from build123d import *

# Parameters (mm, degrees)
SKETCH_1_W          = 131
SKETCH_1_H          = 36
SKETCH_1_W_2        = 125
SKETCH_1_H_2        = 30
EXTRUDE_3_DEPTH     = 50
SKETCH_4_W          = 131
SKETCH_4_H          = 36
EXTRUDE_4_DEPTH     = 3
SKETCH_5_R          = 7.5
CUT_EXTRUDE_1_DEPTH = 3
CUT_EXTRUDE_2_DEPTH = 3
SKETCH_11_W         = 1
SKETCH_11_H         = 30
EXTRUDE_6_DEPTH     = 50
SKETCH_8_W          = 131
SKETCH_8_H          = 36
EXTRUDE_7_DEPTH     = 3
SKETCH_12_W         = 127.4
SKETCH_12_H         = 52.4
CUT_EXTRUDE_4_DEPTH = 3
CUT_EXTRUDE_5_DEPTH = 3
FILLET_5_R          = 3
FILLET_6_R          = 1


with BuildPart() as part:
    # 草图1 → 凸台-拉伸3 (new body)
    with BuildSketch(Plane.XY):
        with Locations((62.5, -15)):
            Rectangle(SKETCH_1_W, SKETCH_1_H)
        with Locations((62.5, -15)):
            Rectangle(SKETCH_1_W_2, SKETCH_1_H_2, mode=Mode.SUBTRACT)
    extrude(amount=EXTRUDE_3_DEPTH)

    # 草图4 → 凸台-拉伸4 (add)
    with BuildSketch(Plane(origin=(0, 0, 0), x_dir=(-1, 0, 0), z_dir=(0, 0, -1))):
        with Locations((-62.5, -15)):
            Rectangle(SKETCH_4_W, SKETCH_4_H)
    extrude(amount=EXTRUDE_4_DEPTH)

    # 草图5 → 切除-拉伸1 (cut)
    with BuildSketch(Plane(origin=(0, 3, 0), x_dir=(1, 0, 0), z_dir=(0, 1, 0))):
        with Locations(Location((17.5, -30, 0), (0, 0, 270))):
            Circle(SKETCH_5_R)
        with Locations(Location((47.5, -30, 0), (0, 0, 270))):
            Circle(SKETCH_5_R)
        with Locations(Location((77.5, -30, 0), (0, 0, 270))):
            Circle(SKETCH_5_R)
        with Locations(Location((107.5, -30, 0), (0, 0, 270))):
            Circle(SKETCH_5_R)
    extrude(amount=-CUT_EXTRUDE_1_DEPTH, mode=Mode.SUBTRACT)

    # 草图6 → 切除-拉伸2 (cut)
    with BuildSketch(Plane.XZ.offset(33)):
        Polygon((10, 25), (10, 27.5), (115, 27.5), (115, 25), (115, 22.5), (10, 22.5), align=None)
    extrude(amount=-CUT_EXTRUDE_2_DEPTH, mode=Mode.SUBTRACT)

    # 草图11 → 凸台-拉伸6 (add)
    with BuildSketch(Plane.XY.offset(50)):
        with Locations((0.5, -15)):
            Rectangle(SKETCH_11_W, SKETCH_11_H)
        with Locations((124.5, -15)):
            Rectangle(SKETCH_11_W, SKETCH_11_H)
    extrude(amount=-EXTRUDE_6_DEPTH)

    # 草图8 → 凸台-拉伸7 (add)
    with BuildSketch(Plane.XY.offset(50)):
        with Locations((62.5, -15)):
            Rectangle(SKETCH_8_W, SKETCH_8_H)
    extrude(amount=EXTRUDE_7_DEPTH)

    # 草图12 → 切除-拉伸4 (cut)
    with BuildSketch(Plane(origin=(0, 3, 0), x_dir=(1, 0, 0), z_dir=(0, 1, 0))):
        with Locations((62.5, -25)):
            Rectangle(SKETCH_12_W, SKETCH_12_H)
    extrude(amount=-CUT_EXTRUDE_4_DEPTH, mode=Mode.SUBTRACT)

    # 草图13 → 切除-拉伸5 (cut)
    with BuildSketch(Plane.XY.offset(53)):
        Polygon((47, -15), (47, -5), (78, -5), (78, -25), (47, -25), align=None)
    extrude(amount=-CUT_EXTRUDE_5_DEPTH, mode=Mode.SUBTRACT)

    # 圆角5
    fillet_5_edges = [part.edges().sort_by_distance(p)[0] for p in [
        (-3, -15, 53),
        (62.5, -33, 53),
        (128, -15, 53),
        (128, -15, -3),
        (62.5, -33, -3),
        (-3, -15, -3),
        (128, -33, 25),
        (-3, -33, 25),
    ]]
    fillet(fillet_5_edges, radius=FILLET_5_R)

    # 圆角6
    fillet_6_edges = [part.edges().sort_by_distance(p)[0] for p in [
        (47, -15, 50),
        (62.5, -5, 50),
        (78, -15, 50),
        (62.5, -25, 50),
        (47, -15, 53),
        (62.5, -25, 53),
        (78, -15, 53),
        (62.5, -5, 53),
    ]]
    fillet(fillet_6_edges, radius=FILLET_6_R)


solid = part.part
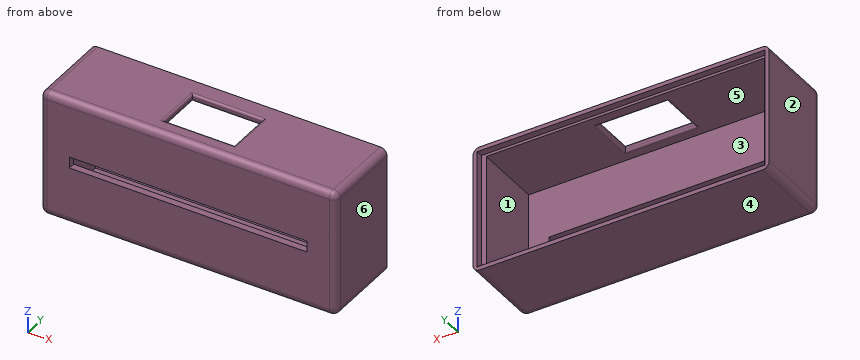
Can you work these out from the model? Positions are in its coordinate system, mm. Face numbers are marked on the shaded views. A direction names the side the tool comes from. Give positions to 0.01 mm unless a question says otherwise; leave off trailing zeros. Order: outer loops, then holes, each group sorted by start corner. A loop starts at its lowest first (then second) coordinate and runs counter-clockwise, first axis right, second up. Notation, with made-up numbers: M -37,48.25 L 14,48.25 A20 cw 14,77.25 Z; hole C 74,-26.75 d8. An arc over 180 degrees is marked long. Use one line per item in the form item = value.
Item 1: If we section it at A-A, the plane x = 64.5: Write out the boundary of the cut face in (y, z).
Values follow:
outline = M -33,0 A3 ccw -30,-3 L 3,-3 L 3,-1.2 L 0,-1.2 L 0,0 L -30,0 L -30,22.5 L -33,22.5 Z; M -33,27.5 L -30,27.5 L -30,50 L -26,50 A1 ccw -25,51 L -25,52 A1 ccw -26,53 L -30,53 A3 ccw -33,50 Z; M -5,51 A1 ccw -4,50 L 0,50 L 0,51.2 L 3,51.2 L 3,53 L -4,53 A1 ccw -5,52 Z
Item 2: For the marked faces 5 and 6, which set-ups out of +Z, -Z, +X, -X, +Y, -Y let a thin tool reach every point of the face, with its end or its side?
Values follow:
face_5 = +Y
face_6 = +Z, -Z, +X, +Y, -Y
Item 3: If we section it at C-C, the plane x = 24: Write out the boundary of the cut face in (y, z).
Values follow:
outline = M -33,0 A3 ccw -30,-3 L 3,-3 L 3,-1.2 L 0,-1.2 L 0,0 L -30,0 L -30,22.5 L -33,22.5 Z; M -33,27.5 L -30,27.5 L -30,50 L 0,50 L 0,51.2 L 3,51.2 L 3,53 L -30,53 A3 ccw -33,50 Z
Item 4: Will these pins go through, and if not, where does the flat tip stop? pin 1 Ø0.9 at (x, y) = (57, -32) entering from +Z; pin 2 Ø15.5 at (x, z) = (91, 37) entering from +Y; pin 3 Ø0.9 at (x, y) = (56.5, -32) entering from -Z.
Values follow:
pin_1 = 52.57
pin_2 = -30
pin_3 = -2.57
Item 5: If I drill on line 1 along Z through (x, y) = (113, -11.5); line 2 along X through (y, z) = (-25, 33); line 3 along Z through (x, y) = (14, 1), over which ranges is the centre line in solid material (lowest first)? Write a range as [from, to].
Values follow:
line_1 = [-3, 0], [50, 53]
line_2 = [-3, 1], [124, 128]
line_3 = [-3, -1.2], [51.2, 53]
Item 6: If we section it at B-B, the plane y = -27.5: Write out the boundary of the cut face in (x, z).
Values follow:
outline = M -3,0 A3 ccw 0,-3 L 125,-3 A3 ccw 128,0 L 128,50 A3 ccw 125,53 L 0,53 A3 ccw -3,50 Z; hole M 1,0 L 124,0 L 124,50 L 1,50 Z
Item 7: Thinking about a two-plate mould opening in X: for the marked faces 1, 2, 3 and 4, which applies, pulls with the +X half, pulls with the -X half, needs draft (parallel to the pull), parting line crosses it, or undercut?
Values follow:
face_1 = undercut
face_2 = pulls with the -X half
face_3 = undercut
face_4 = needs draft
Item 8: If we section it at D-D, the plane z = 1.5: Write out the boundary of the cut face in (x, y).
Values follow:
outline = M -3,-30 A3 ccw 0,-33 L 125,-33 A3 ccw 128,-30 L 128,3 L 126.2,3 L 126.2,0 L 124,0 L 124,-30 L 1,-30 L 1,0 L -1.2,0 L -1.2,3 L -3,3 Z
